The listing builds one solid part. Answer for the finished solid, in the listing's coordinates (mm). Face numbers are marked on the shaded views. A direction names the side the tool comes from. Coordinates: 2 decimals unless noted, no trailing zeros. Loops run counter-clockwise (first coordinate to the right, second up) from the corner with the lowest first, then second, coordinate; pieces in that order, holes last. Notation, with made-up numbers: (84.25, -11.5) -> (123.25, -11.5) arc R11 ccw to (123.25, 0.5) -> close; hole circle Ø4 at (18.25, 37.25). An arc over 180 degrees is marked (long way). Answer in a Markdown table with one row per item.
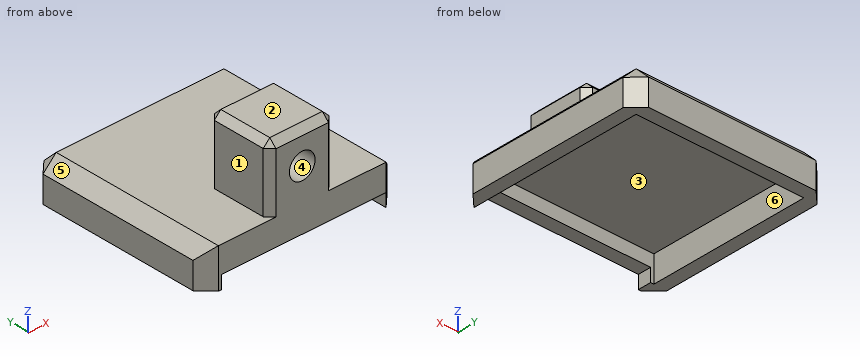
Autodesk Inventor part; units mm, degrees
ref_plane "YZ Plane" through (0, 0, 0) normal (1, 0, 0) x (0, 1, 0)
ref_plane "XZ Plane" through (0, 0, 0) normal (0, 1, 0) x (-1, 0, 0)
ref_plane "XY Plane" through (0, 0, 0) normal (0, 0, 1) x (1, 0, 0)
sketch "Skizze1" plane through (0, 0, 0) normal (0, 0, 1) x (1, 0, 0)
  point P0 (0, 0)
sketch "Skizze2" plane through (0, 0, 0) normal (0, 0, 1) x (1, 0, 0)
  line L0 (-12.75, 12.25) -> (12.75, 12.25)
  line L1 (12.75, 12.25) -> (12.75, -12.25)
  line L2 (12.75, -12.25) -> (-12.75, -12.25)
  line L3 (-12.75, -12.25) -> (-12.75, 12.25)
  line L4 (0, 19.95) -> (0, -19.95)
  line L5 (-20.65, 0) -> (20.65, 0)
  line L6 (-14.75, 14.25) -> (14.75, 14.25)
  line L7 (14.75, 14.25) -> (14.75, -14.25)
  line L8 (14.75, -14.25) -> (-14.75, -14.25)
  line L9 (-14.75, -14.25) -> (-14.75, 14.25)
  point P0 (0, 0)
  dimension "d0" = 25.5
  dimension "d1" = 24.5
  dimension "d2" = 2
  dimension "d3" = 2
  dimension "d4" = 2
  dimension "d5" = 2
extrude "Extrusion1" add sketch "Skizze2" along normal blind 4 contours L3 L5 L9 L6 L4 L0 | L4 L6 L7 L5 L1 L0 | L3 L2 L4 L8 L9 L5 | L5 L7 L8 L4 L2 L1
sketch "Skizze3" plane through (0, 0, 4) normal (0, 0, 1) x (1, 0, 0)
  line L0 (14.75, -14.25) -> (-14.75, -14.25)
  line L1 (-14.75, 14.25) -> (14.75, 14.25)
  line L2 (14.75, 14.25) -> (14.75, -14.25)
  line L3 (14.75, -14.25) -> (-14.75, -14.25)
  line L4 (-14.75, -14.25) -> (-14.75, 14.25)
  point P0 (0, 0)
extrude "Extrusion2" add sketch "Skizze3" along normal blind 2
sketch "Skizze4" plane through (0, 0, 0) normal (0, 0, -1) x (-1, 0, 0)
  line L0 (12.75, -12.25) -> (-12.75, -12.25)
  line L1 (-12.75, -12.25) -> (12.25, -12.25)
  line L2 (12.25, -12.25) -> (12.25, -17.2138)
  line L3 (12.25, -17.2138) -> (-12.75, -17.2138)
  line L4 (-12.75, -17.2138) -> (-12.75, -12.25)
  point P0 (0, 0)
extrude "Extrusion3" cut sketch "Skizze4" against normal blind 2
sketch "Skizze5" plane through (0, 0, 0) normal (0, 0, -1) x (-1, 0, 0)
  circle A0 centre (0.25, 13.25) radius 0.5
  line L0 (14.75, 14.25) -> (-14.75, 14.25)
  line L1 (14.75, -14.25) -> (14.75, 14.25)
  line L2 (-14.75, 14.25) -> (-14.75, -14.25)
  circle A1 centre (-9.75, 13.25) radius 0.5
  circle A2 centre (10.25, 13.25) radius 0.5
  circle A3 centre (-13.75, 0.25) radius 0.5
  circle A4 centre (-13.75, -9.75) radius 0.5
  circle A5 centre (-13.75, 10.25) radius 0.5
  line L3 (0, -19.95) -> (0, 19.95)
  circle A6 centre (13.75, 0.25) radius 0.5
  circle A7 centre (13.75, -9.75) radius 0.5
  circle A8 centre (13.75, 10.25) radius 0.5
  point P0 (0, 0)
  point P1 (13.75, 14.25)
  point P2 (-13.75, 14.25)
  point P3 (14.75, -13.25)
  point P4 (14.75, 13.25)
  point P5 (-14.75, 13.25)
  point P6 (-14.75, -13.25)
  dimension "d15" = 1
  dimension "d16" = 1
  dimension "d17" = 1
  dimension "d18" = 1
  dimension "d19" = 10
  dimension "d20" = 10
  dimension "d21" = 1
  dimension "d22" = 1
  dimension "d23" = 1
  dimension "d24" = 1
  dimension "d25" = 10
  dimension "d26" = 10
sketch "Skizze6" plane through (0, 0, 6) normal (0, 0, 1) x (1, 0, 0)
  line L0 (-5, -4.25) -> (5, -4.25)
  line L1 (5, -4.25) -> (5, -14.25)
  line L2 (5, -14.25) -> (-5, -14.25)
  line L3 (-5, -14.25) -> (-5, -4.25)
  line L4 (0, 19.95) -> (0, -19.95)
  line L5 (-20.65, 0) -> (20.65, 0)
  line L6 (-13.75, -14.25) -> (13.75, -14.25)
  point P0 (0, 0)
  dimension "d29" = 10
  dimension "d30" = 10
  dimension "d59" = 0
extrude "Extrusion5" add sketch "Skizze6" along normal blind 10
sketch "Skizze9" plane through (-5, -4.25, 6) normal (0, 1, 0) x (1, 0, 0)
  circle A0 centre (5, -5) radius 1.95
  line L0 (10, -10) -> (0, -10)
  point P0 (5, 6)
  dimension "d52" = 3.9
  dimension "d53" = 5
extrude "Extrusion8" cut sketch "Skizze9" against normal blind 26
chamfer "Fase4" distance 1 angle 45 8 edges at (-5, -9.25, 16) (0, -14.25, 16) (5, -14.25, 11) (5, -4.25, 11) (0, -4.25, 16) (-5, -4.25, 11) (-5, -14.25, 11) (5, -9.25, 16)
chamfer "Fase5" distance 2 angle 45 7 edges at (14.75, -14.25, 3) (14.75, 0, 6) (0, 14.25, 6) (-14.75, 0, 6) (-14.75, -14.25, 3) (-14.75, 14.25, 3) (14.75, 14.25, 3)
properties part number "20181106_Raspberrycamhalter"
Item 1: A cutting plane is placed at B-B, the plane z = 3.5. Determine the outline of the cut face in (x, y), plus the area to 3 significant figures.
Findings below:
| item | result |
|---|---|
| outline | (-14.75, -12.25) -> (-12.75, -14.25) -> (12.75, -14.25) -> (14.75, -12.25) -> (14.75, 12.25) -> (12.75, 14.25) -> (-12.75, 14.25) -> (-14.75, 12.25) -> close; hole (-12.75, -12.25) -> (12.75, -12.25) -> (12.75, 12.25) -> (-12.75, 12.25) -> close |
| area | 208 mm2 |
Item 2: A tool of negligible diameter and unlimited length cuts with its end or side. For the marked faces 5 and 6, from which of +Z, -Z, +X, -X, +Y, -Y can it reach the whole face along a straight path? Write none if from no direction.
Findings below:
| item | result |
|---|---|
| face 5 | +Z, -X, +Y, -Y |
| face 6 | -Z |
Item 3: Find the intervals of material crossed by probe 1 along Z at (x, y) = (0, -11); probe 2 along X at (y, z) = (-7.25, 11); probe 3 along Z at (x, y) = (-11.5, 12), in increasing order.
Findings below:
| item | result |
|---|---|
| probe 1 | z = 4 to 9.05, 12.95 to 16 |
| probe 2 | x = -5 to -1.95, 1.95 to 5 |
| probe 3 | z = 4 to 6 |
Item 4: Determine the mould class of the marked faces 1, 2, 3 and 4 for opening direction X: +X half, -X half, draft (parallel to the pull), parting line (faces both ways), or undercut.
Findings below:
| item | result |
|---|---|
| face 1 | -X half |
| face 2 | draft |
| face 3 | undercut |
| face 4 | undercut |
Item 5: A cutting plane is placed at D-D, the plane z = 11. Determine the outline of the cut face in (x, y).
Findings below:
| item | result |
|---|---|
| outline | (-5, -13.25) -> (-4, -14.25) -> (-1.95, -14.25) -> (-1.95, -4.25) -> (-4, -4.25) -> (-5, -5.25) -> close; (1.95, -14.25) -> (4, -14.25) -> (5, -13.25) -> (5, -5.25) -> (4, -4.25) -> (1.95, -4.25) -> close |
Item 6: Flat-ended cylindrical pins translate along their axes: pin 1 Ø1 at (x, y) = (10.5, 8.5) entering from +Z; pin 2 Ø9 at (y, z) = (-7.5, 12) entering from -X; pin 3 Ø1 at (x, y) = (-3, -13) entering from -Z. Find the tip coordinate at first contact, or state that the pin passes through.
Findings below:
| item | result |
|---|---|
| pin 1 | stops at z = 6 |
| pin 2 | stops at x = -5 |
| pin 3 | stops at z = 2 |
Item 7: A cutting plane is placed at A-A, the plane x = 0. Determine the outline of the cut face in (y, z), plus the area to 3 significant figures.
Findings below:
| item | result |
|---|---|
| outline | (-14.25, 2) -> (-12.25, 2) -> (-12.25, 4) -> (12.25, 4) -> (12.25, 0) -> (14.25, 0) -> (14.25, 4) -> (12.25, 6) -> (-4.25, 6) -> (-4.25, 9.05) -> (-14.25, 9.05) -> close; (-14.25, 12.95) -> (-4.25, 12.95) -> (-4.25, 15) -> (-5.25, 16) -> (-13.25, 16) -> (-14.25, 15) -> close |
| area | 127 mm2 |
Item 8: A cutting plane is placed at C-C, the plane z = 8. Determine the outline of the cut face in (x, y), plus the area to 3 significant figures.
Findings below:
| item | result |
|---|---|
| outline | (-5, -13.25) -> (-4, -14.25) -> (4, -14.25) -> (5, -13.25) -> (5, -5.25) -> (4, -4.25) -> (-4, -4.25) -> (-5, -5.25) -> close |
| area | 98.0 mm2 |
